Design review of the part shown in the three views and the two pictorial views. Dimensions are in mm from the part's minimum x, y and z. A direction names the side the tool comes from. Round coordinates to 2 decimals unless told otherwise and drop trailing zeros. Order: outer loops, then holes, each group sorted by start corner. A loop starts at its lowest first (then second) coordinate and runs counter-clockwise, first axis right, second up. Notation, with made-up numbers: (-21, 24) - (7, 24) arc R14 ccw to (7, 28) - close; hole circle Ø5 at (82.25, 73). An arc over 180 degrees is marked (long way). Use CSV: the item, a comma, the result in double quotes.
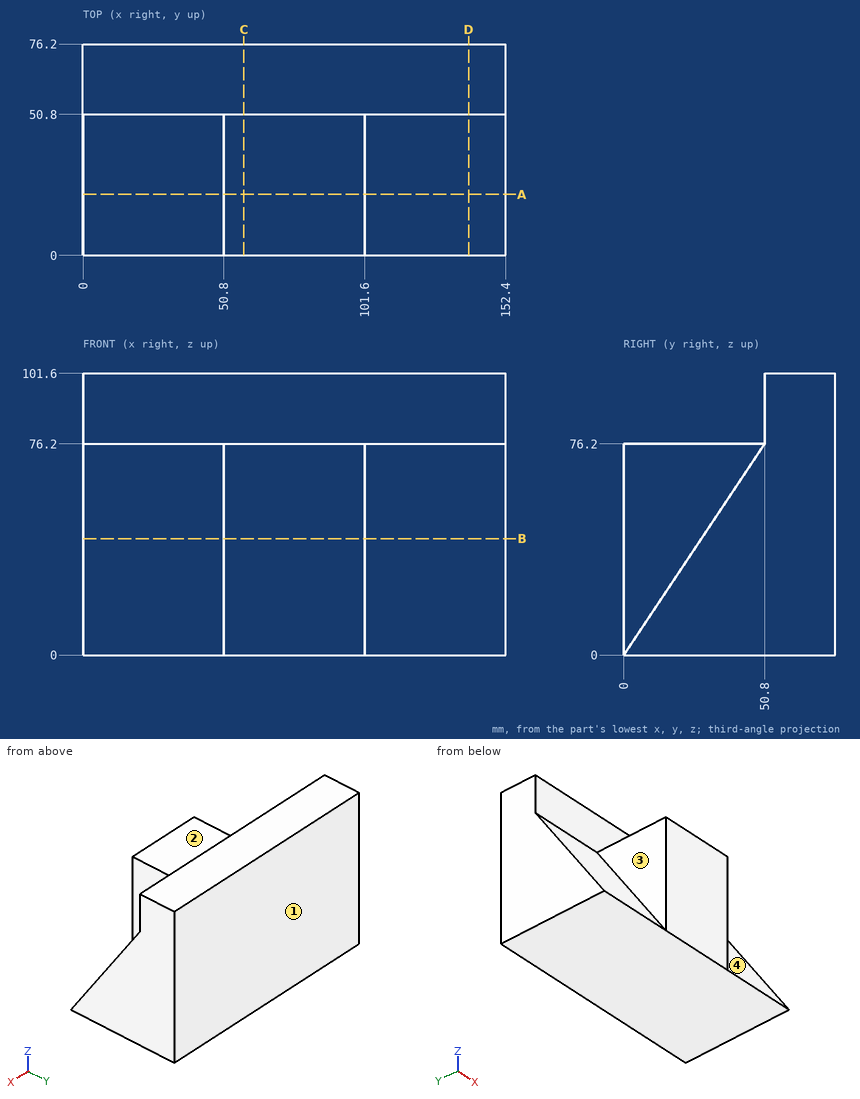
1) We need section B-B (z = 42). Give the boundary of the cut face in (x, y).
Data:
outline,"(0, 28) - (50.8, 28) - (50.8, 0) - (101.6, 0) - (101.6, 28) - (152.4, 28) - (152.4, 76.2) - (0, 76.2) - close"
2) We need section D-D (x = 139). Give the boundary of the cut face in (y, z), then the cut area to 3 significant figures.
Data:
outline,"(0, 0) - (76.2, 0) - (76.2, 101.6) - (50.8, 101.6) - (50.8, 76.2) - close"
area,"4,520 mm2"
3) To check wall thickness, follow L1, parallel to Y at x = 18, z = 81; L2, parallel to Z at x = 92, y = 43; L3, parallel to X at y = 27.5, z = 50.5. State the ranges of each line that lie inside material, in increasing order. Write a range as from..to.
Data:
L1,"y = 50.8..76.2"
L2,"z = 0..76.2"
L3,"x = 50.8..101.6"
4) We need section C-C (x = 58). Give the boundary of the cut face in (y, z).
Data:
outline,"(0, 0) - (76.2, 0) - (76.2, 101.6) - (50.8, 101.6) - (50.8, 76.2) - (0, 76.2) - close"
5) We need section A-A (y = 22). Give the boundary of the cut face in (x, z).
Data:
outline,"(0, 0) - (152.4, 0) - (152.4, 33) - (101.6, 33) - (101.6, 76.2) - (50.8, 76.2) - (50.8, 33) - (0, 33) - close"
6) Insertion check: pin 1 Ø15 at (x, y) = (85.5, 35) entering from +Z; pin 2 Ø20.5 at (x, z) = (59.5, 90) entering from -Y. Each pin has a flat end and moves straight along its axis. Give the tip position at first contact, or say it passes through.
Data:
pin 1,"stops at z = 76.2"
pin 2,"stops at y = 50.8"
7) For the marked faces 1, 2, 3 and 4, list the 3-axis set-ups (+Z, -Z, +X, -X, +Y, -Y) from which the entire face can be reached by the end or side of a thin tool; tool diameter is ignored.
Data:
face 1,"+Z, -Z, +X, -X, +Y"
face 2,"+Z, +X, -X, -Y"
face 3,"+Z, -X, -Y"
face 4,"+Z, +X, -Y"
